from build123d import *

# Parameters (mm, degrees)
F1_DEPTH = 100


with BuildPart() as f1:
    # F0 (on Top) → F1 (new body)
    with BuildSketch(Plane.XY):
        with BuildLine():
            Line((0, 75), (0, 0))
            Line((0, 0), (50, 0))
            Line((50, 0), (50, 12.5))
            ThreePointArc((50, 12.5), (25, 37.5), (50, 62.5))
            Line((50, 62.5), (50, 75))
            Line((50, 75), (0, 75))
        make_face()
        with BuildLine():
            Line((50, 12.5), (50, 0))
            ThreePointArc((50, 0), (87.5, 37.5), (50, 75))
            Line((50, 75), (50, 62.5))
            ThreePointArc((50, 62.5), (67.67767, 55.17767), (75, 37.5))
            ThreePointArc((75, 37.5), (67.67767, 19.82233), (50, 12.5))
        make_face()
    extrude(amount=F1_DEPTH)


solid = f1.part
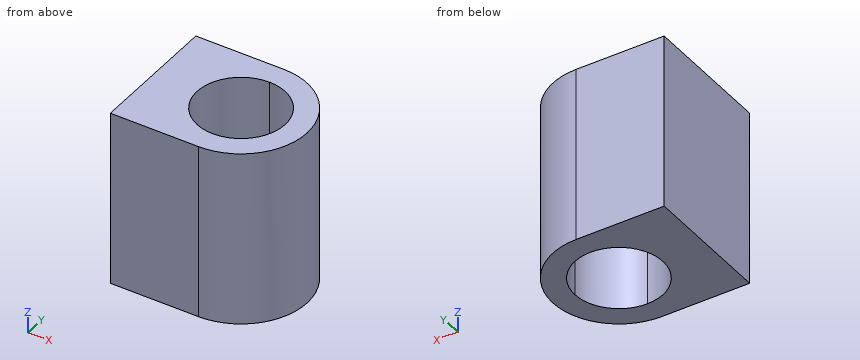
Design review of the part built by this model. Coordinates are the model's own, in mm. Coordinates: 2 decimals unless noted, no trailing zeros. Order: outer loops, then holes, each group sorted by start corner. A loop starts at its lowest first (then second) coordinate and runs counter-clockwise, first axis right, second up. Notation, with made-up numbers: M 47,-12.5 L 100,-12.5 A27 ccw 100,19.5 Z; hole C 1.25,89 d3. An arc over 180 degrees is marked long. Use a Markdown table: item, result.
(1) Add section B-B (y = 45). Give the boundary of the cut face in (x, z).
Worked answers:
| item | result |
|---|---|
| outline | M 0,0 L 26.15,0 L 26.15,100 L 0,100 Z; M 73.85,0 L 86.74,0 L 86.74,100 L 73.85,100 Z |
(2) Add section C-C (x = 59). Give the boundary of the cut face in (y, z).
Worked answers:
| item | result |
|---|---|
| outline | M 1.1,0 L 14.18,0 L 14.18,100 L 1.1,100 Z; M 60.82,0 L 73.9,0 L 73.9,100 L 60.82,100 Z |
(3) Wall thickness on probe 1 along X at (y, z) = (21.5, 75); probe 2 along Y at (x, z) = (34.5, 89.5); probe 3 along X at (y, z) = (32.5, 83.5): over which ranges is each line inside the solid? List them lowest first.
Worked answers:
| item | result |
|---|---|
| probe 1 | x = 0 to 30.79, 69.21 to 83.92 |
| probe 2 | y = 0 to 17.88, 57.12 to 75 |
| probe 3 | x = 0 to 25.51, 74.49 to 87.17 |
(4) Add section D-D (x = 80). Give the boundary of the cut face in (y, z), then the cut area to 3 significant figures.
Worked answers:
| item | result |
|---|---|
| outline | M 15,0 L 60,0 L 60,100 L 15,100 Z |
| area | 4,500 mm2 |
(5) Add section A-A (z = 54). Give the boundary of the cut face in (x, y).
Worked answers:
| item | result |
|---|---|
| outline | M 0,0 L 50,0 A37.5 ccw 50,75 L 0,75 Z; hole M 50,12.5 A25 ccw 75,37.5 A25 ccw 50,62.5 A25 ccw Z |
(6) For P1, Ø1, axis at y = 32, z = 47, coming from the +X side; P2, Ø2, axis at x = 74, z = 70, coming from the -Y side; P3, Ø3, axis at y = 59, z = 40.5, coming from the +X side, all flat-tipped, find the tip position at first contact; note any pin that passes through.
Worked answers:
| item | result |
|---|---|
| P1 | stops at x = 87.17 |
| P2 | stops at y = 7.88 |
| P3 | stops at x = 81.72 |
